Autodesk Inventor part; units mm, degrees
ref_plane "YZ Plane" through (0, 0, 0) normal (1, 0, 0) x (0, 1, 0)
ref_plane "XZ Plane" through (0, 0, 0) normal (0, 1, 0) x (-1, 0, 0)
ref_plane "XY Plane" through (0, 0, 0) normal (0, 0, 1) x (1, 0, 0)
sketch "Sketch1" plane through (0, 0, 0) normal (0, 1, 0) x (-1, 0, 0)
  line L0 (0, 0) -> (-17, 0)
  line L1 (-17, 0) -> (-17, -3)
  line L2 (-17, -3) -> (0, -3)
  line L3 (0, -3) -> (0, 0)
  line L4 (0, 0) -> (3, 0)
  line L5 (3, 0) -> (3, -20)
  line L6 (3, -20) -> (0, -20)
  line L7 (0, -20) -> (0, 0)
  dimension "d0" = 3
  dimension "d1" = 3
  dimension "d3" = 20
  dimension "d56" = 20
extrude "Extrusion1" add sketch "Sketch1" along normal blind 35
fillet "Fillet1" radius 2 1 edges at (0, 17.5, -3)
fillet "Fillet2" radius 5 1 edges at (-3, 17.5, 0)
sketch "Sketch3" plane through (17, 0, -3) normal (0, 0, -1) x (1, 0, 0)
  line L0 (0, -35) -> (-15, -35)
  line L1 (-15, 0) -> (0, 0)
  line L2 (0, 0) -> (0, -35)
  point P0 (-17, 0)
  point P1 (-7.5, -27.5)
  point P2 (-17, 35)
  point P3 (-17, 0)
  point P4 (-7.5, -7.5)
  point P5 (-17, -35)
  dimension "d21" = 7.5
  dimension "d57" = 7.5
  dimension "d58" = 7.5
hole "Hole2" at (9.5, 27.5, -3) at (9.5, 7.5, -3) direction (0, 0, 1) diameter 4.5 end through all
sketch "Sketch4" plane through (-3, 0, -20) normal (-1, 0, 0) x (0, 0, 1)
  line L0 (15, 35) -> (5, 54.5)
  line L1 (5, 54.5) -> (-10, 54.5)
  line L2 (-10, 54.5) -> (-10, 19.5)
  line L3 (0, 0) -> (0, 35)
  line L4 (-10, 19.5) -> (0, 0)
  line L5 (5, 54.5) -> (-10, 54.5)
  line L6 (-10, 54.5) -> (-10, 59.5)
  line L7 (-10, 59.5) -> (5, 59.5)
  line L8 (5, 59.5) -> (5, 54.5)
  line L9 (20, 0) -> (20, 35)
  line L10 (17, 25.25) -> (17, 29.75)
  line L11 (20, 29.75) -> (20, 25.25)
  line L12 (17, 25.25) -> (17, 29.75)
  line L13 (0, 35) -> (15, 35)
  dimension "d30" = 5
  dimension "d32" = 15
  dimension "d34" = 15
  dimension "d59" = 19.5
extrude "Extrusion2" add sketch "Sketch4" against normal up to surface (3 mm away)
sketch "Sketch5" plane through (-3, 19.5, -30) normal (-1, 0, 0) x (0, 0, 1)
  line L0 (10, -19.5) -> (25, -19.5)
  line L1 (0, 40) -> (0, 0)
  line L2 (15, 40) -> (0, 40)
  line L3 (0, 40) -> (0, 37)
  line L4 (0, 37) -> (15, 37)
  line L5 (15, 37) -> (15, 40)
  line L6 (25, 15.5) -> (15, 35)
  line L7 (15, 35) -> (15, 40)
  line L8 (15, 40) -> (0, 40)
  line L9 (0, 40) -> (0, 0)
  line L10 (0, 0) -> (10, -19.5)
  line L11 (25, 15.5) -> (25, -19.5)
  point P0 (30, -19.5)
  dimension "d52" = 3
  dimension "d53" = 15
extrude "Extrusion3" add sketch "Sketch5" against normal blind 23 contours L1 L2 L5 L4
fillet "Fillet3" radius 2 1 edges at (0, 56.5, -22.5)
fillet "Fillet4" radius 5 1 edges at (-3, 59.5, -22.5)
sketch "Sketch6" plane through (22, 59.5, -15) normal (0, 1, 0) x (-1, 0, 0)
  line L0 (2, -15) -> (2, 0)
  point P0 (9.5, -7.5)
  point P1 (2, -7.5)
  point P2 (2, -7.5)
  dimension "d54" = 7.5
hole "Hole3" at (12.5, 59.5, -22.5) direction (0, -1, 0) diameter 4.5 end through all
sketch "Sketch7" plane through (-3, 0, -20) normal (-1, 0, 0) x (0, 0, 1)
  line L0 (-10, 54.5) -> (5, 54.5)
  line L1 (-10, 54.5) -> (-10, 19.5)
  point P0 (20, 0)
  point P1 (2, 39.5)
  dimension "d60" = 15
  dimension "d61" = 12
hole "Hole4" at (-3, 39.5, -18) direction (1, 0, 0) diameter 3 end through all
chamfer "Chamfer1" distance 0.5 angle 45 2 edges at (-3, 39.5, -19.5) (0, 39.5, -19.5)
equation "\"d1\" = d0"
properties part number "Top_Angle Bracket Small" material "Aluminum 6061"
Work out the finished part from the listing and answer in its coordinate system (mm). A direction names the side the tool comes from. Round coordinates to 2 decimals unless told otherwise and drop trailing zeros. Loops run counter-clockwise (first coordinate to the right, second up) from the corner with the lowest first, then second, coordinate; pieces in that order, holes last. Notation, with made-up numbers: M -13.5,56 L -7.5,56 A25 cw -7.5,88 Z; hole C -20,-1 d10. An arc over 180 degrees is marked long. Use CSV: the item, a comma, the result in double quotes.
Q1. Section D-D, the plane x = 13.25 is taken. Determine the outline of the cut face in (y, z).
Determined:
outline,"M 0,-3 L 35,-3 L 35,0 L 0,0 Z; M 56.5,-30 L 59.5,-30 L 59.5,-24.62 L 56.5,-24.62 Z; M 56.5,-20.38 L 59.5,-20.38 L 59.5,-15 L 56.5,-15 Z"
Q2. Section A-A, the plane x = 6 is taken. Determine the outline of the cut face in (y, z).
Determined:
outline,"M 0,-3 L 35,-3 L 35,0 L 0,0 Z; M 56.5,-30 L 59.5,-30 L 59.5,-15 L 56.5,-15 Z"
Q3. Section B-B, the plane y = 27.5 is taken. Determine the outline of the cut face in (x, z), then the cut area to 3 significant figures.
Determined:
outline,"M -3,-30 L 0,-30 L 0,-5 A2 cw 2,-3 L 7.25,-3 L 7.25,0 L 2,0 A5 ccw -3,-5 Z; M 11.75,-3 L 17,-3 L 17,0 L 11.75,0 Z"
area,"123 mm2"
Q4. Section C-C, the plane z = -18 is taken. Determine the outline of the cut face in (x, y), then the cut area to 3 significant figures.
Determined:
outline,"M -3,0 L 0,0 L 0,37.5 L -0.5,38 L -2.5,38 L -3,37.5 Z; M -3,41.5 L -2.5,41 L -0.5,41 L 0,41.5 L 0,54.5 A2 cw 2,56.5 L 20,56.5 L 20,59.5 L 2,59.5 A5 ccw -3,54.5 Z"
area,"224 mm2"
Q5. Consider L1, parallel to X at y = 17, z = -15.75; L2, parallel to Y at x = 11.75, z = -26.5; L3, parallel to X at y = 7.5, z = -1.55. Determine where each line is inside the solid, lowest interval first.
Determined:
L1,"-3 to 0"
L2,"56.5 to 59.5"
L3,"-1.62 to 7.25, 11.75 to 17"
Q6. A tool of negligible diameter and unlimited length cuts with its end or side. For faces 1 (the flat face through (0, 27, -18)), 2 (the flat face through (20, 58, -23)), 3 (the flat face through (7, 35, -2)), from which of +Z, -Z, +X, -X, +Y, -Y can it reach the whole face along a straight path? Write none if from no direction.
Determined:
face 1,"-Z, +X, -Y"
face 2,"+Z, -Z, +X, +Y, -Y"
face 3,"+Z, +X, -X, +Y"
Q7. Each of these flat-tipped pins is pushed along its axis until it touches: pin 1 (6 mm diameter, centred on x = 14.5, z = -19, fed in from -Y); pin 2 (12 mm diameter, centred on x = 12, y = 21, fed in from -Z); pin 3 (3.5 mm diameter, centred on y = 20, z = -1, fed in from +X). Where does it stop, or does it pass through?
Determined:
pin 1,"y = 56.5"
pin 2,"z = -3"
pin 3,"x = 17"
Q8. The mould has two halves that part along X. Classify faces 4 (the flat face through (-1, 44, -30)), 5 (the cylindrical face through (-1.5, 58.07, -22.4)), 6 (the cylindrical face through (7.27, 7.21, -1.48)), 7 (the cylindrical face through (7.603, 28.71, -1.479)): pulls with the +X half, pulls with the -X half, needs draft (parallel to the pull), parting line crosses it, or undercut.
Determined:
face 4,"needs draft"
face 5,"pulls with the -X half"
face 6,"undercut"
face 7,"undercut"
